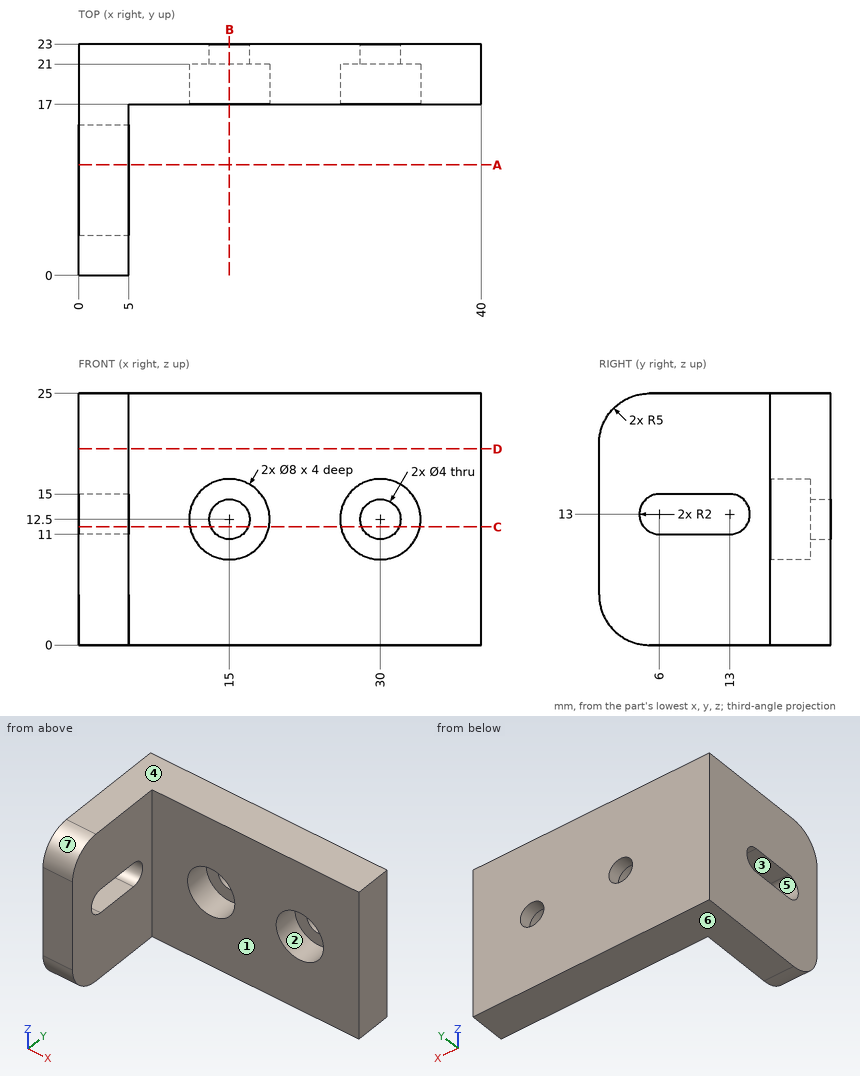
Design review of the part shown in the three views and the two pictorial views. Dimensions are in mm from the part's minimum x, y and z. A direction names the side the tool comes from. Give positions to 0.01 mm unless a question says otherwise; leave off trailing zeros. Loops run counter-clockwise (first coordinate to the right, second up) from the corner with the lowest first, then second, coordinate; pieces in that order, holes last. Notation, with made-up numbers: (-13, 60.25) -> (9, 60.25) arc R14 cw to (9, 76.25) -> close; hole circle Ø8 at (22, -40). An arc over 180 degrees is marked (long way). One line per question, with ' | ' between items.
1) We need section D-D (z = 19.5). Write out the cut boundary in (x, y).
Resolved:
outline: (0, 0) -> (5, 0) -> (5, 17) -> (40, 17) -> (40, 23) -> (0, 23) -> close
2) To check wall thickness, follow probe 1 along Z at (x, y) = (30, 20.25); probe 2 along Z at (x, y) = (3, 11.25); probe 3 along X at (y, z) = (19.25, 16). State the ranges of each line that lie inside material, in increasing order.
Resolved:
probe 1: z = 0 to 8.5, 16.5 to 25 | probe 2: z = 0 to 11, 15 to 25 | probe 3: x = 0 to 13.06, 16.94 to 28.06, 31.94 to 40
3) For the marked faces 1, 2, 3 and 4, list the 3-axis set-ups (+Z, -Z, +X, -X, +Y, -Y) from which the entire face can be reached by the end or side of a thin tool; tool diameter is ignored.
Resolved:
face 1: +Z, -Z, +X, -Y | face 2: -Y | face 3: +X, -X | face 4: +Z, +X, -X, +Y, -Y
4) We need section A-A (y = 11). Write out the cut boundary in (x, z), plus the area to 3 significant figures.
Resolved:
outline: (0, 0) -> (5, 0) -> (5, 11) -> (0, 11) -> close; (0, 15) -> (5, 15) -> (5, 25) -> (0, 25) -> close | area: 105 mm2
5) We need section B-B (x = 15). Write out the cut boundary in (y, z), plus the area to 3 significant figures.
Resolved:
outline: (17, 0) -> (23, 0) -> (23, 10.5) -> (21, 10.5) -> (21, 8.5) -> (17, 8.5) -> close; (17, 16.5) -> (21, 16.5) -> (21, 14.5) -> (23, 14.5) -> (23, 25) -> (17, 25) -> close | area: 110 mm2
6) The part is to be moulded in two halves that separate along Y. For the marked faces 5, 6 and 7, say which applies: +Y half, -Y half, draft (parallel to the pull), parting line (faces both ways), or undercut.
Resolved:
face 5: undercut | face 6: draft | face 7: -Y half
7) We need section C-C (z = 11.75). Write out the cut boundary in (x, y).
Resolved:
outline: (0, 0) -> (5, 0) -> (5, 4.44) -> (0, 4.44) -> close; (0, 14.56) -> (5, 14.56) -> (5, 17) -> (11.07, 17) -> (11.07, 21) -> (13.15, 21) -> (13.15, 23) -> (0, 23) -> close; (16.85, 21) -> (18.93, 21) -> (18.93, 17) -> (26.07, 17) -> (26.07, 21) -> (28.15, 21) -> (28.15, 23) -> (16.85, 23) -> close; (31.85, 21) -> (33.93, 21) -> (33.93, 17) -> (40, 17) -> (40, 23) -> (31.85, 23) -> close
8) Insertion check: pin 1 Ø12 at (y, z) = (7.5, 14) entering from -X; pin 2 Ø8 at (x, z) = (13.5, 21) entering from -Y; pin 3 Ø7 at (x, z) = (30, 12.5) entering from -Y; pin 4 Ø2.5 at (x, z) = (15, 12.5) entering from -Y. Each pin has a flat end and moves straight along its axis. Give the tip position at first contact, or say it passes through.
Resolved:
pin 1: stops at x = 0 | pin 2: stops at y = 17 | pin 3: stops at y = 21 | pin 4: passes through
